Study the drawing (mm; zero at the part's minimum x, y, z) and answer. A direction names the side the tool comes from. Round coordinates to 2 decimals unless told otherwise and drop trailing zeros. Loops run counter-clockwise (first coordinate to the right, second up) from the corner with the lowest first, then second, coordinate; pieces in that order, holes last. Notation, with made-up numbers: M 64.25,-20 L 118.25,-20 A27 ccw 118.25,18 Z; hole C 85.5,17 d7. An arc over 180 degrees is marked long. Put each result on its own line as item: value. Start each with the question number.
(1) Section B-B, the plane z = 4.5 is taken. Determine the outline of the cut face in (x, y).
(2) Determine the mould class of the marked faces 1, 2 and 3 for opening direction X: released by +X, released by -X, zero draft, split by the parting line, or undercut.
(3) Straight lines are drawn through the part: line 1 (Y direction, x = 3.5, z = 5.5); line 2 (Z direction, x = 3.5, y = 22); line 3 (X direction, y = 20, z = 6). For each, find the intervals that lie inside material, in ascending order.
(4) Section C-C, the plane x = 3.5 is taken. Determine the outline of the cut face in (y, z).
(5) Which of the six approach directions +Z, -Z, +X, -X, +Y, -Y give full straight-line access (tool end or side, diameter ignored) to the marked faces 4, 5 and 6?
(6) Section D-D, the plane z = 9 is taken. Determine the outline of the cut face in (x, y), then the cut area to 3 significant figures.
(7) Flat-ended cylindrical pins translate along their axes: P1, Ø2, axis at x = 5.5, y = 14, coming from the -Z side; P2, Ø1.5, axis at y = 34.5, z = 4, coming from the +X side; P3, Ø1.5, axis at x = 2, z = 8.5, coming from the +Y side. Find the tip coordinate at first contact, or state that the pin passes through.
(8) Section A-A, the plane y = 3.5 is taken. Determine the outline of the cut face in (x, z).
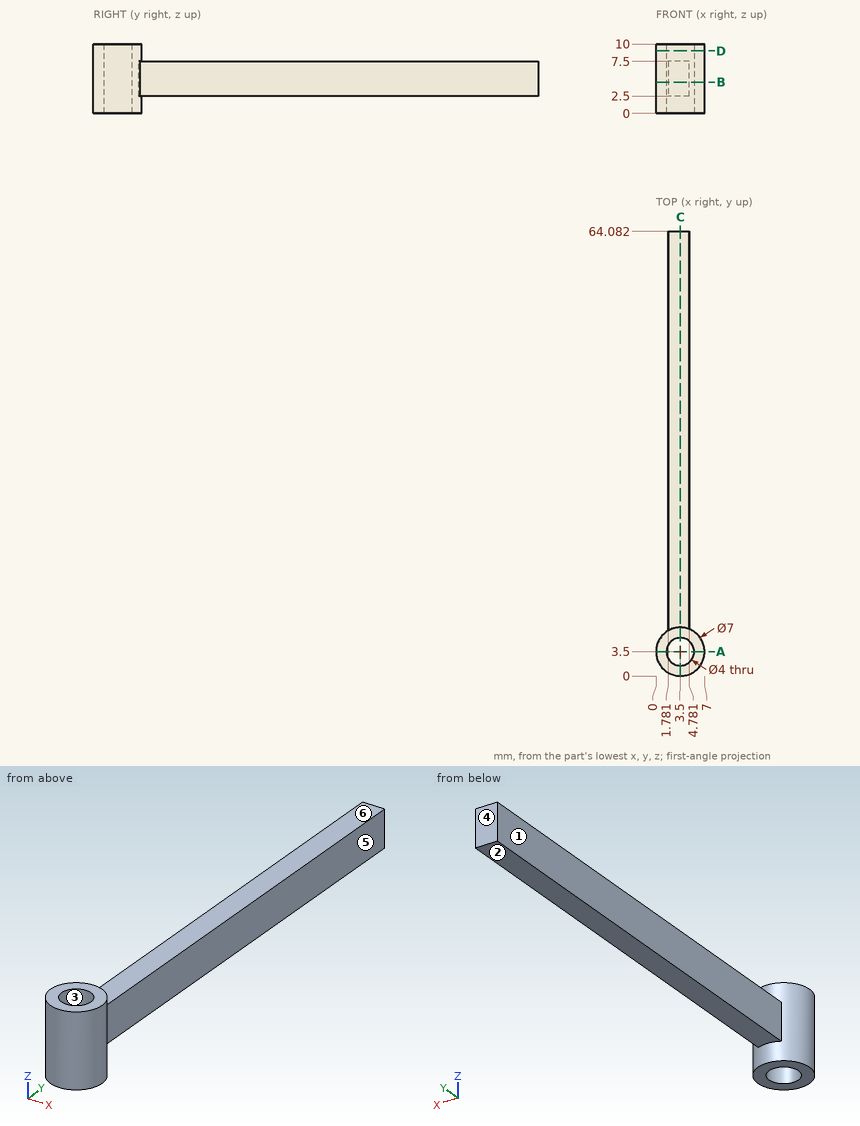
Recorded:
1. outline: M 1.78,6.55 A3.5 ccw long 4.78,6.76 L 4.78,64.08 L 1.78,64.08 Z; hole C 3.5,3.5 d4
2. face 1: released by -X
2. face 2: zero draft
2. face 3: undercut
3. line 1: y = 0 to 1.5, 5.5 to 64.08
3. line 2: z = 2.5 to 7.5
3. line 3: x = 1.78 to 4.78
4. outline: M 0,0 L 1.5,0 L 1.5,10 L 0,10 Z; M 5.5,0 L 7,0 L 7,2.5 L 64.08,2.5 L 64.08,7.5 L 7,7.5 L 7,10 L 5.5,10 Z
5. face 4: +Z, -Z, +X, -X, +Y
5. face 5: +Z, -Z, +X, +Y
5. face 6: +Z, +X, -X, +Y
6. outline: C 3.5,3.5 d7; hole C 3.5,3.5 d4
6. area: 25.9 mm²
7. P1: stops at z = 2.5
7. P2: stops at x = 4.78
7. P3: stops at y = 6.92
8. outline: M 0,0 L 1.5,0 L 1.5,10 L 0,10 Z; M 5.5,0 L 7,0 L 7,10 L 5.5,10 Z
